Autodesk Fusion 360 part; units mm, degrees
sketch "Boceto1" plane through (0, 0, 0) normal (0, 0, 1) x (1, 0, 0)
  line L0 (-5, -7.5) -> (-5, 7.5)
  circle A0 centre (0, 8) radius 2
  line L1 (-6, 0) -> (7, 0) construction
  line L2 (0, 8) -> (0, -7) construction
  line L3 (5, -7.5) -> (5, 7.5)
  arc A1 (5, 7.5) -> (-5, 7.5) centre (0, 7.5) ccw
  arc A2 (-5, -7.5) -> (5, -7.5) centre (0, -7.5) ccw
  point P0 (-5, 0)
  point P1 (5, 0)
  dimension "d7" = 15
  dimension "d11" = 4
  dimension "d13" = 5
  dimension "d15" = 15
  dimension "d16" = 5
extrude "Extruir1" add sketch "Boceto1" along normal blind 3
Verification items for the finished model (mm, model axes). Round coordinates to 2 decimals unless told otherwise and drop trailing zeros. Order: outer loops, then holes, each group sorted by start corner. A loop starts at its lowest first (then second) coordinate and runs counter-clockwise, first axis right, second up.
1) Depth check by flat-ended pin: pin 1 (1.5 mm diameter, centred on x = 1, z = 0.5, fed in from -Y); pin 2 (3 mm diameter, centred on x = 0, y = 8, fed in from +Z). Enter the tip coordinate at first touch or a pass-through.
Geometry says:
pin 1: stops at y = -12.49
pin 2: passes through
2) Material ranges on line 1 (Y direction, x = 0, z = 1.25); line 2 (Y direction, x = 1.5, z = 1.1); line 3 (X direction, y = -9, z = 2.55), recorded low to high.
Geometry says:
line 1: y = -12.5 to 6, 10 to 12.5
line 2: y = -12.27 to 6.68, 9.32 to 12.27
line 3: x = -4.77 to 4.77
3) Cross-section at B-B, the plane y = 9.5. Record the cut outline in (x, z), plus the area to 3 significant figures.
Geometry says:
outline: (-4.58, 0) - (-1.32, 0) - (-1.32, 3) - (-4.58, 3) - close; (1.32, 0) - (4.58, 0) - (4.58, 3) - (1.32, 3) - close
area: 19.6 mm2
4) Draft check along X on faces 1 (the flat face through (-5, 0, 1)), 2 (the flat face through (0, 0, 3)), 3 (the cylindrical face through (0, 6, 1)). Enter one of: +X half, -X half, draft (parallel to the pull), parting line (faces both ways), or undercut.
Geometry says:
face 1: -X half
face 2: draft
face 3: undercut
5) Cross-section at A-A, the plane x = 0. Record the cut outline in (y, z).
Geometry says:
outline: (-12.5, 0) - (6, 0) - (6, 3) - (-12.5, 3) - close; (10, 0) - (12.5, 0) - (12.5, 3) - (10, 3) - close
6) Cross-section at D-D, the plane x = -2.75. Record the cut outline in (y, z), plus the area to 3 significant figures.
Geometry says:
outline: (-11.68, 0) - (11.68, 0) - (11.68, 3) - (-11.68, 3) - close
area: 70.1 mm2
7) Cross-section at C-C, the plane z = 0.7. Record the cut outline in (x, y), plus the area to 3 significant figures.
Geometry says:
outline: (-5, -7.5) arc R5 ccw to (5, -7.5) - (5, 7.5) arc R5 ccw to (-5, 7.5) - close; hole circle Ø4 at (0, 8)
area: 216 mm2
